Input: part model. Units: mm. Frame: model coordinates. Coordinates: 2 decimals unless noted, no trailing zeros. Loops run counter-clockwise (first coordinate to the right, second up) from the corner with the lowest first, then second, coordinate; pieces in that order, holes last. Notation, with made-up numbers: (38, 28.5) - (46, 28.5) arc R21 cw to (46, 33.5) - close; hole circle Ø5 at (5.25, -31.5). An arc over 180 degrees is marked (long way). Use a Markdown table: item, result. Add a question column.
1. Section query B-B on x = 12.5. Return the cut outline in (y, z), then the cut area to 3 significant figures.
2. Ray query, L1, parallel to Z at x = 13, y = -4.5; L2, parallel to Z at x = 78.5, y = -3.75; L3, parallel to X at y = -4.75, z = -90. Return the intervals inside material, ascending. Write a range as [from, to].
3. Section query A-A on x = 63. Return the cut outline in (y, z), then the cut area to 3 significant figures.
4. Section query C-C on z = -127. Return the cut outline in (x, y).
5. Section query D-D on x = 91.5. Return the cut outline in (y, z).
6. Contact query for flat-ended pins moving along their axis: P1, Ø3, axis at x = 17.5, z = -25, coming from the +Y side; P2, Ø2, axis at y = -3.175, z = -96, coming from the +X side; P3, Ø1.5, axis at x = 77.5, y = -4, coming from the -Z side. Output: stop coordinate, or through.
```python
from build123d import *

# Parameters (mm, degrees)
BASE_FLANGE1_DEPTH                   = 6.35
SKETCH8_R                            = 3.4
CUT_EXTRUDE1_DEPTH                   = 183.851914127
SKETCH9_R                            = 18.5
CUT_EXTRUDE2_DEPTH                   = 183.851914127
SKETCH11_R                           = 1.2
CUT_EXTRUDE4_DEPTH                   = 183.851914127
BOSS_EXTRUDE2_START                  = -6.35
BOSS_EXTRUDE2_DEPTH                  = 6.35
TAP_DRILL_FOR_M3X0_5_TAP2_AT_2_COUNT = 2
TAP_DRILL_FOR_M3X0_5_TAP2_AT_2_PITCH = 12
CIRPATTERN3_COUNT                    = 2
CIRPATTERN3_ANGLE                    = 60


# Sheet-metal steps are written as plain solids
with BuildPart() as part:
    # Sketch2 → Base-Flange1 (new body)
    with BuildSketch(Plane(origin=(0, 0, 0), x_dir=(1, 0, 0), z_dir=(0, 1, 0))):
        with BuildLine():
            Line((0, 0), (50.76093065, 0))
            Line((50.76093065, 0), (107.880465325, 57.119534675))
            ThreePointArc((107.880465325, 57.119534675), (111.537953618, 118.761570635), (50.76093065, 129.682710556))
            Line((50.76093065, 129.682710556), (0, 90))
            Line((0, 90), (0, 0))
        make_face()
    extrude(amount=-BASE_FLANGE1_DEPTH)

    # Sketch8 → Cut-Extrude1 (cut, through all)
    with BuildSketch(Plane(origin=(0, 0, 0), x_dir=(1, 0, 0), z_dir=(0, 1, 0))):
        with Locations(Location((12.5, 79, 0), (0, 0, 270))):
            Circle(SKETCH8_R)
        with Locations(Location((12.5, 11, 0), (0, 0, 90))):
            Circle(SKETCH8_R)
    extrude(amount=-CUT_EXTRUDE1_DEPTH, mode=Mode.SUBTRACT)

    # Sketch9 → Cut-Extrude2 (cut, through all)
    with BuildSketch(Plane(origin=(0, 0, 0), x_dir=(1, 0, 0), z_dir=(0, 1, 0))):
        with Locations(Location((75, 90, 0), (0, 0, 270))):
            Circle(SKETCH9_R)
    extrude(amount=-CUT_EXTRUDE2_DEPTH, mode=Mode.SUBTRACT)

    # Sketch11 → Cut-Extrude4 (cut, through all)
    with BuildSketch(Plane(origin=(0, 0, 0), x_dir=(1, 0, 0), z_dir=(0, 1, 0))):
        with Locations(Location((17.5, 25, 0), (0, 0, 270))):
            Circle(SKETCH11_R)
        with Locations(Location((17.5, 34.5, 0), (0, 0, 270))):
            Circle(SKETCH11_R)
    extrude(amount=-CUT_EXTRUDE4_DEPTH, mode=Mode.SUBTRACT)

    # Sketch15 → Boss-Extrude2 (add)
    with BuildSketch(Plane.XZ.offset(6.35).offset(BOSS_EXTRUDE2_START)):
        with BuildLine():
            Line((129, -100), (129, -80))
            ThreePointArc((129, -80), (122.450687881, -77.994187792), (118.147884423, -72.66477373))
            ThreePointArc((118.147884423, -72.66477373), (121.5, -90), (118.147884423, -107.33522627))
            ThreePointArc((118.147884423, -107.33522627), (122.450687881, -102.005812208), (129, -100))
        make_face()
    boss_extrude2 = extrude(amount=BOSS_EXTRUDE2_DEPTH)

    # Sketch17 → Tap Drill for M3x0.5 Tap2 (revolve, cut)
    with BuildSketch(Plane(origin=(129, -3.175, -84), x_dir=(0, 0, -1), z_dir=(0, 1, 0))):
        Polygon((0, 0), (0, 5.751075774), (1.25, 5), (1.25, 0), align=None)
    tap_drill_for_m3x0_5_tap2 = revolve(axis=Axis((135.35, -3.175, -84), (-1, 0, 0)), mode=Mode.SUBTRACT)

    # Tap Drill for M3x0.5 Tap2 at 2: Tap Drill for M3x0.5 Tap2 ×2
    with Locations(*[(0, 0, -i * TAP_DRILL_FOR_M3X0_5_TAP2_AT_2_PITCH) for i in range(1, TAP_DRILL_FOR_M3X0_5_TAP2_AT_2_COUNT)]):
        add(tap_drill_for_m3x0_5_tap2, mode=Mode.SUBTRACT)

    # CirPattern3: Boss-Extrude2, Tap Drill for M3x0.5 Tap2 ×2 about axis
    cirpattern3_axis = Axis((75, 0, -90), (0, 1, 0))
    add([boss_extrude2.rotate(cirpattern3_axis, i * CIRPATTERN3_ANGLE / (CIRPATTERN3_COUNT - 1)) for i in range(1, CIRPATTERN3_COUNT)])
    add([tap_drill_for_m3x0_5_tap2.rotate(cirpattern3_axis, i * CIRPATTERN3_ANGLE / (CIRPATTERN3_COUNT - 1)) for i in range(1, CIRPATTERN3_COUNT)], mode=Mode.SUBTRACT)

    # CirPattern3 copy 1 sketch → CirPattern3 copy 1 (revolve, cut)
    with BuildSketch(Plane(origin=(96.803847577, -3.175, -139.765371804), x_dir=(-0.8660254037844399, 0, -0.4999999999999978), z_dir=(0, 1, 0))):
        Polygon((0, 0), (0, 5.751075774), (1.25, 5), (1.25, 0), align=None)
    revolve(axis=Axis((99.978847577, -3.175, -145.264633118), (-0.4999999999999978, 0, 0.8660254037844399)), mode=Mode.SUBTRACT)


solid = part.part
```
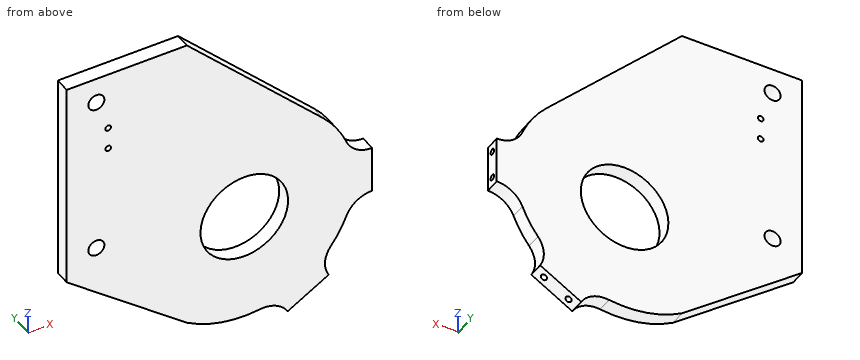
Resolved:
| question | item | result |
|---|---|---|
| 1 | outline | (-6.35, -99.77) - (0, -99.77) - (0, -82.4) - (-6.35, -82.4) - close; (-6.35, -75.6) - (0, -75.6) - (0, -14.4) - (-6.35, -14.4) - close; (-6.35, -7.6) - (0, -7.6) - (0, 0) - (-6.35, 0) - close |
| 1 | area | 547 mm² |
| 2 | L1 | [-100.16, -82.36], [-75.64, -14.36], [-7.64, 0] |
| 2 | L2 | [-136.37, -108.17], [-71.83, -27.74] |
| 2 | L3 | [0, 56.5], [93.5, 129] |
| 3 | outline | (-6.35, -134.92) - (0, -134.92) - (0, -104.08) - (-6.35, -104.08) - close; (-6.35, -75.92) - (0, -75.92) - (0, -12.24) - (-6.35, -12.24) - close |
| 3 | area | 600 mm² |
| 4 | outline | (47.33, -6.35) - (109.14, -6.35) - (109.14, 0) - (47.33, 0) - close |
| 5 | outline | (-6.35, -139.36) - (0, -139.36) - (0, -98.37) - (-6.35, -98.37) - close; (-6.35, -81.63) - (0, -81.63) - (0, -40.74) - (-6.35, -40.74) - close |
| 6 | P1 | y = 0 |
| 6 | P2 | x = 123.85 |
| 6 | P3 | z = -136.47 |
